```python
from build123d import *

# Parameters (mm, degrees)
F0_R     = 20.5
F0_R_2   = 19
F0_W     = 23.9
F0_H     = 23
F2_DEPTH = 14
F1_W     = 23.9
F1_H     = 23
F1_R     = 2.25
F1_R_2   = 8.3
F0_R_3   = 2.25
F0_R_4   = 1.6
F3_DEPTH = 3
F4_R     = 6
F6_DEPTH = 15
F5_W     = 12
F5_H     = 3
F7_DEPTH = 25
F8_DEPTH = 25


with BuildPart() as f2:
    # F0 (on Top) → F2 (new body)
    with BuildSketch(Plane.XY):
        Circle(F0_R)
        Circle(F0_R_2, mode=Mode.SUBTRACT)
        Circle(F0_R_2)
        Rectangle(F0_W, F0_H, mode=Mode.SUBTRACT)
    extrude(amount=F2_DEPTH)

    # F1 (on face) + F0 (on Top) → F3 (join)
    with BuildSketch(Plane.XY):
        Rectangle(F1_W, F1_H)
        with Locations((9.15, -8.7)):
            Circle(F1_R, mode=Mode.SUBTRACT)
        with Locations((1.3, -0.9836626705)):
            Circle(F1_R_2, mode=Mode.SUBTRACT)
        with Locations((-3.15, 8.8)):
            Circle(F1_R, mode=Mode.SUBTRACT)
    with BuildSketch(Plane.XY):
        with Locations((-3.15, 8.8)):
            Circle(F0_R_3)
        with Locations((-3.15, 8.8)):
            Circle(F0_R_4, mode=Mode.SUBTRACT)
        with Locations((9.15, -8.7)):
            Circle(F0_R_3)
        with Locations((9.15, -8.7)):
            Circle(F0_R_4, mode=Mode.SUBTRACT)
        with Locations((-3.15, 8.8)):
            Circle(F0_R_4)
        with Locations((9.15, -8.7)):
            Circle(F0_R_4)
    extrude(amount=F3_DEPTH)

    # F4
    f4_edges = [f2.edges().sort_by_distance(p)[0] for p in [
        (-20.5, 0, 0),
    ]]
    fillet(f4_edges, radius=F4_R)

    # F0 (on Top) → F6 (join)
    with BuildSketch(Plane.XY):
        with Locations((-3.15, 8.8)):
            Circle(F0_R_4)
        with Locations((9.15, -8.7)):
            Circle(F0_R_4)
    extrude(amount=F6_DEPTH)

    # F5 (on Right) → F7 (cut)
    with BuildSketch(Plane.YZ):
        with Locations((-0.6070649059, 6.5)):
            Rectangle(F5_W, F5_H)
    extrude(amount=-F7_DEPTH, mode=Mode.SUBTRACT)

    # F8 (cut): a face of the model
    f8_faces = [f2.faces().sort_by_distance(p)[0] for p in [
        (-16.077019229, -0.5627771714, 8),
    ]]
    extrude(f8_faces, amount=-F8_DEPTH, mode=Mode.SUBTRACT)


solid = f2.part
```
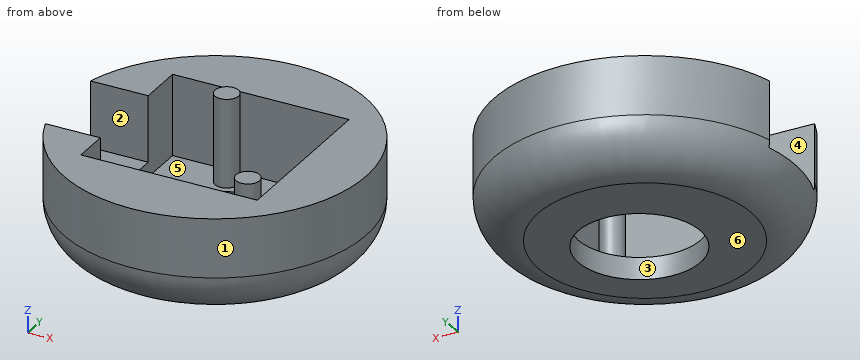
Read the model definition and answer for the solid it produces. Units are mm, in the model's axes. Face numbers are marked on the shaded views. A direction names the side the tool comes from. Coordinates: 2 decimals unless noted, no trailing zeros. Order: outer loops, then holes, each group sorted by start corner. A loop starts at its lowest first (then second) coordinate and runs counter-clockwise, first axis right, second up. Notation, with made-up numbers: (70, 49) - (74, 49) arc R7 ccw to (74, 53) - close; hole circle Ø5 at (87.5, 1.25). An arc over 180 degrees is marked (long way). Answer as a JSON object with one key per item and string values. Group by question number.
Item 1: Flat-ended cylindrical pins translate along their axes: P1, Ø3.5, axis at y = 5.5, z = 7.5, coming from the -X side; P2, Ø5, axis at y = -7, z = 8, coming from the -X side; P3, Ø10, axis at x = 1.3, y = -0.98, coming from the -Z side; P4, Ø3, axis at x = -16, z = 4.5, coming from the +Y side. Find the tip coordinate at first contact, or state that the pin passes through.
Item 2: Section C-C (z = 4.25) is taken. Give the vertices of the cut face in (x, y), plus the area to 3 significant figures.
Item 3: A tool of negligible diameter and unlimited length cuts with its end or side. For the marked faces 4, 5 and 6, from which of +Z, -Z, +X, -X, +Y, -Y can it reach the whole face along a straight path? Write none if from no direction.
Item 4: Section A-A (z = 11) is taken. Give the vertices of the cut face in (x, y), plus the area to 3 significant figures.
Item 5: Consider probe 1 along X at (y, z) = (-9, 13.5); probe 2 along Y at (x, z) = (-3.5, 9.75); probe 3 along X at (y, z) = (8.5, 4.5). Determine where each line is inside the solid, lowest interval first. Write a range as from..to.
Item 6: Section B-B (y = 0) is taken. Give the vertices of the cut face in (x, z).
Item 7: The mould has two halves that part along X. Classify the marked faces 1, 2 and 3: +X half, -X half, draft (parallel to the pull), parting line (faces both ways), or undercut.
Results are:
{
 "1": {"P1": "stops at x = -19.78", "P2": "stops at x = -19.41", "P3": "passes through", "P4": "stops at y = 14.29"},
 "2": {"outline": "circle Ø40.48 at (0, 0); circle Ø3.2 at (-3.15, 8.8); circle Ø3.2 at (9.15, -8.7); hole (-11.95, -11.5) - (11.95, -11.5) - (11.95, 11.5) - (-11.95, 11.5) - close", "area": "753 mm^2"},
 "3": {"face 4": "+Z, -X", "face 5": "+Z", "face 6": "-Z, +X, -X, +Y, -Y"},
 "4": {"outline": "(-19.78, 5.39) - (-11.95, 5.39) - (-11.95, 11.5) - (11.95, 11.5) - (11.95, -11.5) - (-11.95, -11.5) - (-11.95, -6.61) - (-19.41, -6.61) arc R20.5 ccw (long way) to start; circle Ø3.2 at (-3.15, 8.8); circle Ø3.2 at (9.15, -8.7)", "area": "688 mm^2"},
 "5": {"probe 1": "x = -18.42..-11.95, 7.58..10.72, 11.95..18.42", "probe 2": "y = -20.2..-11.5, 7.24..10.36, 11.5..20.2", "probe 3": "x = -18.45..-11.95, -4.72..-1.58, 11.95..18.45"},
 "6": {"outline": "(-20.42, 5) arc R6 ccw to (-14.5, 0) - (-6.94, 0) - (-6.94, 3) - (-11.95, 3) - (-11.95, 5) - close; (9.54, 0) - (14.5, 0) arc R6 ccw to (20.5, 6) - (20.5, 14) - (11.95, 14) - (11.95, 3) - (9.54, 3) - close"},
 "7": {"face 1": "parting line", "face 2": "draft", "face 3": "undercut"}
}
